```python
from build123d import *

# Parameters (mm, degrees)
F0_W     = 1370
F0_H     = 115
F1_DEPTH = 9
F2_W     = 1370
F2_H     = 98
F3_DEPTH = 9
F4_SIZE  = 5
F5_SIZE  = 10
F6_SIZE  = 10


with BuildPart() as f1:
    # F0 (on Front) → F1 (new body)
    with BuildSketch(Plane.XZ):
        Rectangle(F0_W, F0_H)
    extrude(amount=F1_DEPTH)

    # F2 (on face) → F3 (join)
    with BuildSketch(Plane.XZ.offset(9)):
        with Locations((0, -8.5)):
            Rectangle(F2_W, F2_H)
    extrude(amount=F3_DEPTH)

    # F4
    f4_edges = [f1.edges().sort_by_distance(p)[0] for p in [
        (0, 0, 57.5),
    ]]
    chamfer(f4_edges, length=F4_SIZE)

    # F5
    f5_edges = [f1.edges().sort_by_distance(p)[0] for p in [
        (685, -7, 57.5),
    ]]
    chamfer(f5_edges, length=F5_SIZE)

    # F6
    f6_edges = [f1.edges().sort_by_distance(p)[0] for p in [
        (-685, -7, 57.5),
    ]]
    chamfer(f6_edges, length=F6_SIZE)


solid = f1.part
```
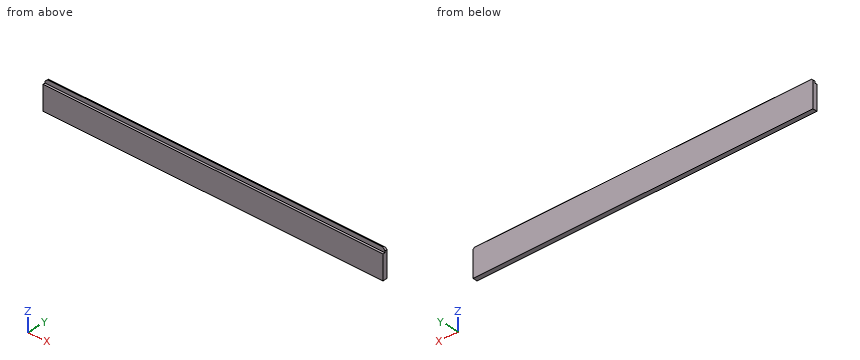
Could you check a few things on this model? Use its own coordinates, in mm. Give positions to 0.01 mm unless a question says otherwise; leave off trailing zeros. Loops run counter-clockwise (first coordinate to the right, second up) from the corner with the lowest first, then second, coordinate; pieces in that order, holes last. Notation, with made-up numbers: (-3, 80.5) - (33, 80.5) arc R22 ccw to (33, 114.5) - close; hole circle Ø6 at (87.25, -10). An arc over 180 degrees is marked (long way). Use one line per item in the form item = value.
1. I want a section at A-A (x = -534.5). Please give me the cut outline in (y, z), and give its area (3 significant figures).
Response values:
outline = (-18, -57.5) - (0, -57.5) - (0, 52.5) - (-5, 57.5) - (-9, 57.5) - (-9, 40.5) - (-18, 40.5) - close
area = 1,900 mm²
2. I'm going to push flat-ended pins straight in: pin 1 Ø8.5 at (x, z) = (104.5, 49.5) entering from -Y; pin 2 Ø1 at (x, y) = (187.5, -3) entering from +Z; pin 3 Ø7 at (x, y) = (171.5, -14.5) entering from +Z. Where does each tip first touch, or does it pass through?
Response values:
pin_1 = -9
pin_2 = 56
pin_3 = 40.5
3. I need wall thicknesses on probe 1 along Y at (x, z) = (-165.5, 45); probe 2 along Z at (x, y) = (543, -12.5); probe 3 along Z at (x, y) = (-7.5, -4). Which ranges of each line are inside material? Lowest first, please.
Response values:
probe_1 = -9 to 0
probe_2 = -57.5 to 40.5
probe_3 = -57.5 to 56.5
